Autodesk Inventor part; units mm, degrees
ref_plane "YZ Plane" through (0, 0, 0) normal (1, 0, 0) x (0, 1, 0)
ref_plane "XZ Plane" through (0, 0, 0) normal (0, 1, 0) x (-1, 0, 0)
ref_plane "XY Plane" through (0, 0, 0) normal (0, 0, 1) x (1, 0, 0)
sketch "Sketch1" plane through (0, 0, 0) normal (0, 0, 1) x (1, 0, 0)
  line L0 (-10, 15) -> (10, 15)
  line L1 (10, 15) -> (10, -15)
  line L2 (10, -15) -> (-10, -15)
  line L3 (-10, -15) -> (-10, 15)
  line L4 (-10, 15) -> (10, -15) construction
  line L5 (10, 15) -> (-10, -15) construction
  point P0 (0, 0)
  dimension "d0" = 20
  dimension "d1" = 30
extrude "Extrusion1" add sketch "Sketch1" along normal blind 50
shell "Shell1" thickness 3 removed faces 1 at (-3.3333, 5, 50)
sketch "Sketch2" plane through (-10, 15, 0) normal (0, 1, 0) x (1, 0, 0)
  line L0 (3, -3) -> (17, -3)
  line L1 (-7, -47) -> (17, -47)
  line L2 (17, -47) -> (17, -3)
  line L3 (17, -3) -> (-7, -3)
  line L4 (-7, -3) -> (-7, -47)
  line L5 (-7, -47) -> (17, -3) construction
  line L6 (17, -47) -> (-7, -3) construction
  point P0 (10, 0)
  point P1 (5, -25)
sketch "Sketch3" plane through (0, 0, 0) normal (0, 0, -1) x (-1, 0, 0)
  line L0 (-10, 15) -> (10, 15)
  line L1 (10, 15) -> (10, -15)
  line L2 (-10, 15) -> (10, 15)
  line L3 (10, 15) -> (10, 12.5)
  line L4 (10, 12.5) -> (-10, 12.5)
  line L5 (-10, 12.5) -> (-10, 15)
  line L6 (-10, -15) -> (-10, 15)
  line L7 (10, -15) -> (-10, -15)
  line L8 (-10, -15) -> (-10, -12.5)
  line L9 (-10, -12.5) -> (10, -12.5)
  line L10 (10, -12.5) -> (10, -15)
  point P0 (0, 0)
  point P1 (10, -12.5)
  dimension "d5" = 2.5
  dimension "d6" = 2.5
extrude "Extrusion2" add sketch "Sketch3" along normal blind 15 contours L0 L1 L4 L5 | L9 L1 L7 L6
sketch "Sketch4" plane through (-10, 15, 50) normal (0, 1, 0) x (1, 0, 0)
  point P0 (10, 50)
sketch "Sketch6" plane through (-10, -15, 50) normal (0, -1, 0) x (1, 0, 0)
  circle A0 centre (4.0698, -58) radius 1.6
  circle A1 centre (15, -58) radius 1.6
  point P0 (10, -50)
extrude "Extrusion4" cut sketch "Sketch6" against normal through all
fillet "Fillet1" radius 2 4 edges at (-7, -12, 26.5) (10, -15, 17.5) (-10, 15, 17.5) (10, 15, 17.5)
fillet "Fillet2" radius 2 1 edges at (-10, -15, 17.5)
sketch "Sketch7" plane through (8, -15, -15) normal (0, -1, 0) x (1, 0, 0)
  circle A0 centre (-8, 25.9391) radius 2.5
  point P0 (-8, 15)
  dimension "d17" = 5
extrude "Extrusion5" cut sketch "Sketch7" against normal blind 10
sketch "Sketch8" plane through (0, 0, 50) normal (0, 0, 1) x (1, 0, 0)
  line L0 (-10, 12.5) -> (-10, -12.5)
  line L1 (10, -0.5) -> (-10, -0.5)
  line L2 (-10, -0.5) -> (-10, 0.5)
  line L3 (-10, 0.5) -> (10, 0.5)
  line L4 (10, 0.5) -> (10, -0.5)
  line L5 (10, -0.5) -> (-10, 0.5) construction
  line L6 (-10, -0.5) -> (10, 0.5) construction
  point P0 (0, 0)
  dimension "d20" = 1
extrude "Extrusion6" cut sketch "Sketch8" against normal blind 30
sketch "Sketch9" plane through (0, 0, 50) normal (0, 0, 1) x (1, 0, 0)
  line L0 (-7, 0.5) -> (-3.9859, 12)
  line L1 (-7, 12) -> (7, 12)
  line L2 (-3.9859, 12) -> (2.913, 12)
  line L3 (7, 0.5) -> (2.913, 12)
  line L4 (7, -0.5) -> (2.3967, -12.0157)
  line L5 (2.3967, -12.0157) -> (-2.9074, -12.0157)
  line L6 (7, -12) -> (7, 12)
  line L7 (-7, -10) -> (-7, -0.5)
  line L8 (-2.9074, -12.0157) -> (-7, -0.5)
  line L9 (-7, -0.5) -> (7, -0.5)
  line L10 (10, -12.5) -> (10, 12.5)
  line L11 (7, 0.5) -> (-7, 0.5)
  line L12 (10, 12.5) -> (-10, 12.5)
  line L13 (7, -12) -> (-5, -12)
  arc A0 (-7, -10) -> (-5, -12) centre (-5, -10) ccw
  line L14 (-7, 0.5) -> (-7, 12)
  point P0 (0, 0)
  point P1 (2.403, -12)
  point P2 (-2.913, -12)
extrude "Extrusion7" add sketch "Sketch9" against normal blind 30 contours L14 L1 L0 | L3 L1 L6 | L6 L13 L4 | L8 L13 A0 L7
sketch "Sketch10" plane through (10, -12.5, 0) normal (1, 0, 0) x (0, 0, -1)
  line L0 (-20, 12) -> (-50, 12)
  line L1 (-50, 12) -> (-43.1699, 12)
  line L2 (-43.1699, 12) -> (-43.1699, 9.596)
  line L3 (-43.1699, 9.596) -> (-50, 9.596)
  line L4 (-50, 9.596) -> (-50, 12)
  line L5 (-50, 13) -> (-43.1699, 13)
  line L6 (-43.1699, 13) -> (-43.1699, 14.6143)
  line L7 (-43.1699, 14.6143) -> (-50, 14.6143)
  line L8 (-50, 14.6143) -> (-50, 13)
  point P0 (0, 12.5)
extrude "Extrusion8" add sketch "Sketch10" along normal blind 5
sketch "Sketch11" plane through (10, -2.904, 43.1699) normal (0, -1, 0) x (1, 0, 0)
  circle A0 centre (2.6177, 3.2863) radius 1.5609
  point P0 (-10, -43.1699)
extrude "Extrusion9" cut sketch "Sketch11" against normal blind 6.25
mirror "Mirror1" about plane through (0, 0, 0) normal (1, 0, 0) of "Extrusion8", "Extrusion9"
properties part number "SUCTION_EXTENSION1" material "Iron, Gray"
The model under review builds one solid part; all positions refer to its coordinate system, in mm. A direction names the side the tool comes from. Give positions to 0.01 mm unless a question says otherwise; leave off trailing zeros. Order: outer loops, then holes, each group sorted by start corner. A loop starts at its lowest first (then second) coordinate and runs counter-clockwise, first axis right, second up. Notation, with made-up numbers: M -30.5,-15.75 L 14.5,-15.75 A21 ccw 14.5,-5.75 Z; hole C -14,-16 d5. An arc over 180 degrees is marked long. Answer in a Markdown table with one row per item. Add a question column.
1. Machinability: for faces 1 (the flat face through (0, 12.5, -7)), 2 (the flat face through (-5.514, 6.17, 35.21)), 3 (the flat face through (-12, 1, 43.17)), 4 (the flat face through (9, 0.5, 39)), 5 (the cylindrical face through (-6.4, -11.43, 11.38)), which of the approach directions +Z, -Z, +X, -X, +Y, -Y give a long, thin tool a straight path to every point of the face, cutting with its end or side? Answer none if there is none.
2. Add section B-B on x = 0. State the section outline as (y, z) points.
3. Mouldability with a two-part tool opening along Y and no side actions: class faces 6 (the flat face through (11.9, -2.904, 48.1)), 7 (the flat face through (0, 12, 21)), 8 (the flat face through (4.985, 6.17, 35.21)), 9 (the flat face through (12, -2, 43.17)) as released by +Y, released by -Y, zero draft, split by the parting line, or undercut.
4. For pin 1 Ø2.5 at (x, z) = (-13.5, 45.5) entering from -Y; pin 2 Ø4 at (x, y) = (-10.5, -5) entering from +Z; pin 3 Ø2 at (x, y) = (6, 6) entering from -Z; pin 4 Ø8 at (y, z) = (-5.5, 21.5) entering from -X, all flat-tipped, find the tip position at first contact; note any pin that passes through.
5. Add section D-D on x = 11.75. State the section outline as (y, z) points.
6. Add section A-A on z = -8. State the section outline as (x, y) points, plus the area to 3 significant figures.
7. To check wall thickness, follow line 1 along Y through (x, z) = (1.25, 28); line 2 along X through (y, z) = (2.5, 7.5); line 3 along Z through (x, y) = (-6.75, 4.75). State the ranges of each line that lie inside material, in increasing order.
8. Add section C-C on z = 26.5. State the section outline as (x, y) points, plus the area to 3 significant figures.
The answers:
| question | item | result |
|---|---|---|
| 1 | face 1 | -Z, +X, -X |
| 1 | face 2 | +Z |
| 1 | face 3 | -Z, -X, +Y, -Y |
| 1 | face 4 | +Z, +X, -X |
| 1 | face 5 | none |
| 2 | outline | M -15,-15 L -12.5,-15 L -12.5,0 L 12.5,0 L 12.5,-15 L 15,-15 L 15,50 L 12,50 L 12,3 L -12,3 L -12,8.44 L -15,8.44 Z; M -15,13.44 L -12,13.44 L -12,50 L -15,50 Z |
| 3 | face 6 | released by -Y |
| 3 | face 7 | undercut |
| 3 | face 8 | undercut |
| 3 | face 9 | zero draft |
| 4 | pin 1 | y = -2.9 |
| 4 | pin 2 | z = 50 |
| 4 | pin 3 | z = 0 |
| 4 | pin 4 | x = -10 |
| 5 | outline | M -2.9,43.17 L -0.5,43.17 L -0.5,45.16 L -2.9,45.16 Z; M -2.9,47.75 L -0.5,47.75 L -0.5,50 L -2.9,50 Z; M 0.5,43.17 L 2.11,43.17 L 2.11,45.16 L 0.5,45.16 Z; M 0.5,47.75 L 2.11,47.75 L 2.11,50 L 0.5,50 Z |
| 6 | outline | M -10,-13 A2 ccw -8,-15 L -7.53,-15 L -7.53,-12.5 L -10,-12.5 Z; M -10,12.5 L -7.53,12.5 L -7.53,15 L -8,15 A2 ccw -10,13 Z; M -4.33,-15 L 3.4,-15 L 3.4,-12.5 L -4.33,-12.5 Z; M -4.33,12.5 L 3.4,12.5 L 3.4,15 L -4.33,15 Z; M 6.6,-15 L 8,-15 A2 ccw 10,-13 L 10,-12.5 L 6.6,-12.5 Z; M 6.6,12.5 L 10,12.5 L 10,13 A2 ccw 8,15 L 6.6,15 Z |
| 6 | area | 64.6 mm2 |
| 7 | line 1 | -15 to -12, 12 to 15 |
| 7 | line 2 | -10 to -7, 7 to 10 |
| 7 | line 3 | 0 to 3, 20 to 50 |
| 8 | outline | M -10,-13 A2 ccw -8,-15 L 8,-15 A2 ccw 10,-13 L 10,-0.5 L 7,-0.5 L 2.4,-12 L -2.91,-12 L -7,-0.5 L -10,-0.5 Z; M -10,0.5 L -7,0.5 L -3.99,12 L 2.91,12 L 7,0.5 L 10,0.5 L 10,13 A2 ccw 8,15 L -8,15 A2 ccw -10,13 Z |
| 8 | area | 345 mm2 |
